The listing builds one solid part. Answer for the finished solid, in the listing's coordinates (mm). Face numbers are marked on the shaded views. Give positions to 0.01 mm unless a question says otherwise; leave off trailing zeros. Order: outer loops, then holes, each group sorted by start corner. A loop starts at its lowest first (then second) coordinate and runs counter-clockwise, first axis right, second up. Notation, with made-up numbers: M -34.75,29.5 L -15.75,29.5 A23 ccw -15.75,50.5 Z; hole C 36.5,18.25 d4. An arc over 180 degrees is marked long. Answer as a JSON object with one key per item and string values. Group by question number.
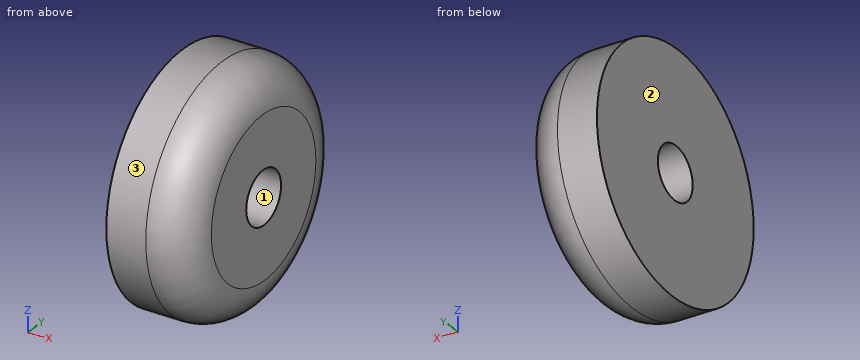
Autodesk Inventor part; units mm, degrees
ref_plane "YZ Plane" through (0, 0, 0) normal (1, 0, 0) x (0, 1, 0)
ref_plane "XZ Plane" through (0, 0, 0) normal (0, 1, 0) x (-1, 0, 0)
ref_plane "XY Plane" through (0, 0, 0) normal (0, 0, 1) x (1, 0, 0)
sketch "Sketch1" plane through (0, 0, 0) normal (1, 0, 0) x (0, 1, 0)
  circle A0 centre (0, 0) radius 4
  circle A1 centre (0, 0) radius 4.5
  dimension "d0" = 8
  dimension "d1" = 0.5
extrude "Extrusion1" add sketch "Sketch1" along normal blind 3 contours A0 | A1
sketch "Sketch2" plane through (3, 0, 0) normal (1, 0, 0) x (0, 0, -1)
  circle A0 centre (0, 0) radius 4.5 construction
hole "Hole1" at (3, 0, 0) direction (-1, 0, 0) diameter 2 depth 8
fillet "Fillet1" radius 1.5 1 edges at (3, -4.5, 0)
properties part number "_3DPrint"
Item 1: Determine the mould class of the marked faces 1, 2 and 3 for opening direction Z: released by +Z, released by -Z, zero draft, split by the parting line, or undercut.
Item 2: Consider probe 1 along Z at (x, y) = (0.65, 0); probe 2 along Y at (x, z) = (1.35, 0.25); probe 3 along Z at (x, y) = (1.25, 3.5). Determine where each line is inside the solid, lowest interval first. Write a range as from..to.
Item 3: A flat-ended cylindrical pin translates along its axis: P1, Ø1, axis at x = 1.5, z = 1, coming from the +Y side. Find the tip coordinate at first contact, or state that the pin passes through.
Item 4: Section A-A (y = 0) is taken. Determine the outline of the cut face in (x, z), and give its area (3 significant figures).
Item 5: Section C-C (x = 0.55) is taken. Determine the outline of the cut face in (y, z), and give its area (3 significant figures).
Values found:
{
 "1": {"face 1": "undercut", "face 2": "zero draft", "face 3": "split by the parting line"},
 "2": {"probe 1": "z = -4.5..-1, 1..4.5", "probe 2": "y = -4.49..-0.97, 0.97..4.49", "probe 3": "z = -2.83..2.83"},
 "3": {"P1": "stops at y = 4.47"},
 "4": {"outline": "M 0,-4.5 L 1.5,-4.5 A1.5 ccw 3,-3 L 3,-1 L 0,-1 Z; M 0,1 L 3,1 L 3,3 A1.5 ccw 1.5,4.5 L 0,4.5 Z", "area": "20.0 mm^2"},
 "5": {"outline": "C 0,0 d9; hole C 0,0 d2", "area": "60.5 mm^2"}
}
